Input: part model. Units: mm. Frame: model coordinates. A direction names the side the tool comes from. Coordinates: 2 decimals unless noted, no trailing zeros. Order: outer loops, then holes, each group sorted by start corner. A loop starts at its lowest first (then second) coordinate and runs counter-clockwise, first axis right, second up.
from build123d import *

# Parameters (mm, degrees)
CROQUIS1_R              = 75
SALIENTE_EXTRUIR1_DEPTH = 20
CROQUIS2_R              = 10
CORTAR_EXTRUIR1_DEPTH   = 10
CORTAR_EXTRUIR2_START   = -10
CROQUIS3_R              = 75
CROQUIS3_R_2            = 35
CORTAR_EXTRUIR2_DEPTH   = 10
CROQUIS4_R              = 5
SALIENTE_EXTRUIR3_DEPTH = 10
CORTAR_EXTRUIR3_START   = -10
CORTAR_EXTRUIR3_DEPTH   = 10


with BuildPart() as part:
    # Croquis1 → Saliente-Extruir1 (new body)
    with BuildSketch(Plane.XY):
        Circle(CROQUIS1_R)
    extrude(amount=SALIENTE_EXTRUIR1_DEPTH)

    # Croquis2 → Cortar-Extruir1 (cut)
    with BuildSketch(Plane.XY.offset(20)):
        Circle(CROQUIS2_R)
    extrude(amount=-CORTAR_EXTRUIR1_DEPTH, mode=Mode.SUBTRACT)

    # Croquis3 → Cortar-Extruir2 (cut)
    with BuildSketch(Plane.XY.offset(20).offset(CORTAR_EXTRUIR2_START)):
        Circle(CROQUIS3_R)
        Circle(CROQUIS3_R_2, mode=Mode.SUBTRACT)
    extrude(amount=CORTAR_EXTRUIR2_DEPTH, mode=Mode.SUBTRACT)

    # Croquis4 → Saliente-Extruir3 (add)
    with BuildSketch(Plane.XY.offset(10)):
        with Locations((50, 0)):
            Circle(CROQUIS4_R)
    extrude(amount=SALIENTE_EXTRUIR3_DEPTH)

    # Croquis5 → Cortar-Extruir3 (cut)
    with BuildSketch(Plane.XY.offset(20).offset(CORTAR_EXTRUIR3_START)):
        with BuildLine():
            ThreePointArc((20, 28.722813233), (15, 0), (20, -28.722813233))
            ThreePointArc((20, -28.722813233), (35, 0), (20, 28.722813233))
        make_face()
    extrude(amount=CORTAR_EXTRUIR3_DEPTH, mode=Mode.SUBTRACT)


solid = part.part
Item 1: Cut plane C-C on y = 0. Return loops of the section in (x, z), then the cut area to 3 significant figures.
Response values:
outline: (-75, 0) - (75, 0) - (75, 10) - (55, 10) - (55, 20) - (45, 20) - (45, 10) - (15, 10) - (15, 20) - (10, 20) - (10, 10) - (-10, 10) - (-10, 20) - (-35, 20) - (-35, 10) - (-75, 10) - close
area: 1,900 mm2
Item 2: Ray query, probe 1 along Y at (x, z) = (0, 13); probe 2 along X at (y, z) = (2.5, 18.75); probe 3 along Z at (x, y) = (-41.5, 42). Return the intervals inside material, ascending.
Response values:
probe 1: y = -35 to -10, 10 to 35
probe 2: x = -34.91 to -9.68, 9.68 to 15.04, 45.67 to 54.33
probe 3: z = 0 to 10
Item 3: Cut plane B-B on x = 0. Return loops of the section in (y, z).
Response values:
outline: (-75, 0) - (75, 0) - (75, 10) - (35, 10) - (35, 20) - (10, 20) - (10, 10) - (-10, 10) - (-10, 20) - (-35, 20) - (-35, 10) - (-75, 10) - close
Item 4: Cut plane D-D on z = 2.25. Return loops of the section in (x, y).
Response values:
outline: circle Ø150 at (0, 0)
Item 5: Pin query (flat end, axial travel): pin 1 Ø5 at (x, z) = (60, 3.5) entering from +Y; pin 2 Ø16 at (x, y) = (0, 0) entering from +Z; pin 3 Ø8 at (y, z) = (20.5, 3) entering from +X. Return the tip coordinate at first contact, or that it passes through.
Response values:
pin 1: stops at y = 48.15
pin 2: stops at z = 10
pin 3: stops at x = 73.16
Item 6: Cut plane A-A on z = 13. Return loops of the section in (x, y).
Response values:
outline: (20, -28.72) arc R85 cw to (20, 28.72) arc R35 ccw (long way) to start; circle Ø10 at (50, 0); hole circle Ø20 at (0, 0)
Item 7: Draft query along X for faces 3 (the face through (-1, 1, 0)), 4 (the face through (45, 0, 15)), 5 (the face through (-9.764, 74.362, 4.93)). Return one class per face: pulls with the +X half, pulls with the -X half, needs draft (parallel to the pull), parting line crosses it, or undercut.
Response values:
face 3: needs draft
face 4: undercut
face 5: parting line crosses it
Item 8: Access query for faces 1 (the face through (-14, 0, 20)), 2 (the face through (-2.17, -9.76, 15.07)). Directions: +Z, -Z, +X, -X, +Y, -Y. A direction counts if a zero-diameter tool reaches every point of the face in a straight line with its end or side. Return the directions, or none.
Response values:
face 1: +Z, +X, -X, +Y, -Y
face 2: +Z
